The model under review builds one solid part; all positions refer to its coordinate system, in mm. Give positions to 0.01 mm unless a question says otherwise; leave off trailing zeros. Order: outer loops, then holes, each group sorted by start corner. A loop starts at its lowest first (then second) coordinate and runs counter-clockwise, first axis right, second up.
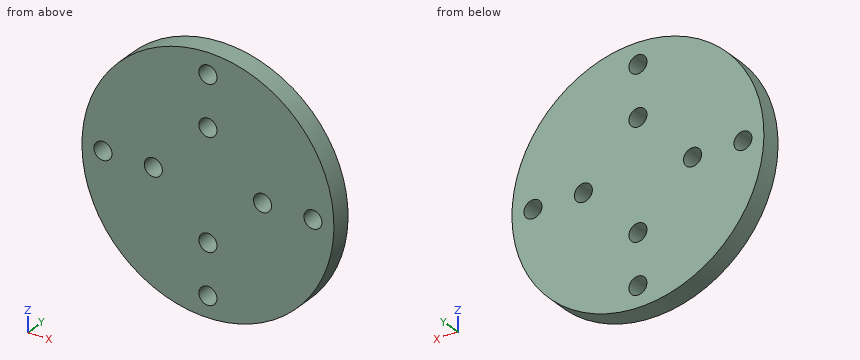
```python
from build123d import *

# Parameters (mm, degrees)
SKETCH1_R            = 30
BOSS_EXTRUDE1_DEPTH  = 5
M4_CLEARANCE_HOLE1_D = 4.3
M4_CLEARANCE_HOLE2_D = 4.3


with BuildPart() as part:
    # Sketch1 → Boss-Extrude1 (new body)
    with BuildSketch(Plane(origin=(0, 0, 0), x_dir=(1, 0, 0), z_dir=(0, 1, 0))):
        with Locations(Location((0, 0, 0), (0, 0, 270))):
            Circle(SKETCH1_R)
    extrude(amount=BOSS_EXTRUDE1_DEPTH)

    # M4 Clearance Hole1 (through all)
    with Locations(Plane(origin=(0, 5, 0), x_dir=(1, 0, 0), z_dir=(0, 1, 0))):
        with Locations((0, -25), (-25, 0), (25, 0), (0, 25)):
            Hole(M4_CLEARANCE_HOLE1_D / 2)

    # M4 Clearance Hole2 (through all)
    with Locations(Plane(origin=(0, 5, 0), x_dir=(1, 0, 0), z_dir=(0, 1, 0))):
        with Locations((-13, 0), (13, 0), (0, 13), (0, -13)):
            Hole(M4_CLEARANCE_HOLE2_D / 2)


solid = part.part
```
1. Take a section at B-B (z = -25). Write out the cut boundary in (x, y).
2. Insertion check: pin 1 (4 mm diameter, centred on x = 0, z = -13, fed in from -Y). The pin has a flat end and moves straight along its axis. Give the tip position at first contact, or say it passes through.
3. To check wall thickness, follow line 1 (X direction, y = 1.1, z = -26.5); line 2 (Z direction, x = -12.5, y = 2.45); line 3 (X direction, y = 1.6, z = 25.5). State the ranges of each line that lie inside material, in increasing order.
4. Take a section at A-A (y = 2.05). Count the separate pieces of the cut face and the enclosed holes in it, and give its area (3 significant figures).
5. Take a section at D-D (x = -14). Write out the cut boundary in (y, z).
6. Take a section at C-C (x = -1). Write out the cut boundary in (y, z), and give its area (3 significant figures).
Answer:
1. outline: (-16.58, 0) - (-2.15, 0) - (-2.15, 5) - (-16.58, 5) - close; (2.15, 0) - (16.58, 0) - (16.58, 5) - (2.15, 5) - close
2. pin 1: passes through
3. line 1: x = -14.06 to -1.54, 1.54 to 14.06
3. line 2: z = -27.27 to -2.09, 2.09 to 27.27
3. line 3: x = -15.8 to -2.09, 2.09 to 15.8
4. separate pieces: 1
4. enclosed holes: 8
4. area: 2,710 mm2
5. outline: (0, -26.53) - (5, -26.53) - (5, -1.9) - (0, -1.9) - close; (0, 1.9) - (5, 1.9) - (5, 26.53) - (0, 26.53) - close
6. outline: (0, -29.98) - (5, -29.98) - (5, -26.9) - (0, -26.9) - close; (0, -23.1) - (5, -23.1) - (5, -14.9) - (0, -14.9) - close; (0, -11.1) - (5, -11.1) - (5, 11.1) - (0, 11.1) - close; (0, 14.9) - (5, 14.9) - (5, 23.1) - (0, 23.1) - close; (0, 26.9) - (5, 26.9) - (5, 29.98) - (0, 29.98) - close
6. area: 224 mm2
